Could you check a few things on this model? Use its own coordinates, in mm. A direction names the side the tool comes from. Round coordinates to 2 decimals unless told otherwise and drop trailing zeros. Write each loop counter-clockwise with the first axis right and the second up, starting at its lowest first coordinate (ties: lowest second). Pieces come first, ordered by that corner, then holes. Notation, with made-up numbers: (51, 41) -> (98, 41) arc R16 ccw to (98, 61) -> close; hole circle Ø3 at (62, -27). An arc over 180 degrees is marked (long way). Answer as CSV lines item,"result". Start each with the question number.
Q1. Imagine slicing it at D-D on y = -3.4. Please give me the cut outline in (x, z), and give its area (3 significant figures).
Q2. Imagine slicing it at B-B on x = -4.5. Please give me the cut outline in (y, z).
Q3. Imagine slicing it at C-C on z = -4.75. Please give me the cut outline in (x, y), and give its area (3 significant figures).
Q4. If we mould it in two halves opening along Z, with no side actions, what happens to faces 1 (the cylindrical face through (-1.544, -2.014, 0.06)), 2 (the flat face through (5, 0, 0)), 3 (the flat face through (6, -2, 2.621))? For each: pulls with the +Z half, pulls with the -Z half, needs draft (parallel to the pull), parting line crosses it, or undercut.
Q5. Imagine slicing it at A-A on y = -2.5. Please give me the cut outline in (x, z), and give its area (3 significant figures).
Q6. For faces 4 (the flat face through (-3.478, -2, -4)), 5 (the cylindrical face through (-3.18, -0.29, -4.34)), 6 (the cylindrical face through (-2.5, -0.3, -1.6)), 7 (the flat face through (-2.64, -1.99, -1.35)), which set-ups out of +Z, -Z, +X, -X, +Y, -Y let a thin tool reach every point of the face, with its end or its side?
Q7. Will these pins go through, and if not, where does the flat tip stop? pin 1 Ø2 at (x, y) = (4.5, -0.5) entering from -Z; pin 2 Ø1 at (y, z) = (-2, -5) entering from -X; pin 3 Ø3 at (x, z) = (-1.5, -1.5) entering from -Y; pin 4 Ø1 at (y, z) = (-0.5, -4.5) entering from +X.
Q8. If I drill on line 1 (Z direction, x = -1.75, y = -0.85); line 2 (Z direction, x = -4.5, y = -2.55); line 3 (Z direction, x = -3.25, y = -2.1), over which ranges is the centre line in solid material (lowest first)? Write a range as [from, to].
from build123d import *

# Parameters (mm, degrees)
F1_DEPTH = 4
F2_R     = 0.75
F3_R     = 1


with BuildPart() as f1:
    # F0 (on Front) → F1 (new body)
    with BuildSketch(Plane.XZ):
        Polygon((-3.4779643061, -6.6976709247), (16.9765876419, 2.6205155937), (-6.205236799, 2.6205155937), (-6.205236799, 0.575057485), (0.1584017682, 0.575057485), (-3.4779643061, -1.924942515), align=None)
    extrude(amount=F1_DEPTH)

    # F2
    f2_edges = [f1.edges().sort_by_distance(p)[0] for p in [
        (0.158402, -2, 0.575057),
    ]]
    fillet(f2_edges, radius=F2_R)

    # F3
    f3_edges = [f1.edges().sort_by_distance(p)[0] for p in [
        (-3.477964, -4, -4.311307),
        (-2.654714, -4, -1.358958),
        (-3.477964, 0, -4.311307),
        (-1.540112, 0, 0.047517),
    ]]
    fillet(f3_edges, radius=F3_R)


solid = f1.part
Checks:
1,outline,"(-6.21, 0.66) -> (-2.26, 0.66) arc R0.83 cw to (-1.78, -0.86) -> (-3.39, -1.97) -> (-3.39, -6.66) -> (16.98, 2.62) -> (-6.21, 2.62) -> close"
1,area,"96.4 mm^2"
2,outline,"(-4, 1.58) arc R1 ccw to (-3, 0.58) -> (-1, 0.58) arc R1 ccw to (0, 1.58) -> (0, 2.62) -> (-4, 2.62) -> close"
3,outline,"(-3.48, -3) arc R1 ccw to (-2.48, -4) -> (0.8, -4) -> (0.8, 0) -> (-2.48, 0) arc R1 ccw to (-3.48, -1) -> close"
3,area,"16.7 mm^2"
4,face 1,"undercut"
4,face 2,"needs draft"
4,face 3,"pulls with the +Z half"
5,outline,"(-6.21, 0.58) -> (-2.26, 0.58) arc R0.75 cw to (-1.83, -0.79) -> (-3.48, -1.92) -> (-3.48, -6.7) -> (16.98, 2.62) -> (-6.21, 2.62) -> close"
5,area,"97.4 mm^2"
6,face 4,"-Z, -X, +Y, -Y"
6,face 5,"-Z, -X, +Y"
6,face 6,"-X, +Y"
6,face 7,"-X, +Y, -Y"
7,pin 1,"z = -3.52"
7,pin 2,"x = -3.48"
7,pin 3,"y = -4"
7,pin 4,"x = 2.44"
8,line 1,"[-5.91, -0.74], [0.39, 2.62]"
8,line 2,"[0.58, 2.62]"
8,line 3,"[-6.59, -1.77], [0.58, 2.62]"
